Input: part model. Units: mm. Frame: model coordinates. A direction names the side the tool comes from. Coordinates: 2 decimals unless noted, no trailing zeros. Write each loop counter-clockwise with the first axis right and the second up, starting at its lowest first coordinate (ties: lowest second). Pieces come first, ordered by that corner, then holes. Notation, with made-up numbers: M 12.25,63.25 L 69.25,63.25 A20 ccw 69.25,70.25 Z; hole C 61.5,-2 d10. An arc over 180 degrees is marked long. Write each question's results on one line, items separated by ' | '. Start each with the question number.
1. First-contact query: pin 1 (10 mm diameter, centred on y = -29, z = 8, fed in from +X); pin 2 (5 mm diameter, centred on y = -5, z = 15.5, fed in from -X); pin 3 (4.5 mm diameter, centred on y = -5, z = -15.5, fed in from +X); pin 4 (14.5 mm diameter, centred on x = 0, z = 0, fed in from +Y). Flat tips, straight axial feed; report the tip coordinate or a pass-through.
2. Section query A-A, the plane y = 2.5. Count the separate pieces of the cut face and the enclosed holes in it, and give its area (3 significant figures).
3. Section query C-C, the plane y = -27. Output: boundary loops of the cut face in (x, z), and give its area (3 significant figures).
4. Section query B-B, the plane z = -6.5. Output: boundary loops of the cut face in (x, y), and give its area (3 significant figures).
5. Set-up query: faces 5 (the flat face through (-23.85, -30, -15)), 6 (the cylindrical face through (-24.8, -26.5, -14.7)). Return all of +Z, -Z, +X, -X, +Y, -Y with unobstructed straight access to the full face (end or side cutting, diameter ignored); none if empty.
6. Pull-direction query (Y, two-part tool) for faces 1 (the flat face through (-13, 5, 0)), 2 (the flat face through (-2.73, -16.6, -23.96)), 3 (the flat face through (-23.85, -5, -17.5)), 4 (the flat face through (-21, -16, 0)); classes: +Y half, -Y half, draft (parallel to the pull), parting line (faces both ways), or undercut.
7. Section query D-D, the plane x = 0. Output: boundary loops of the cut face in (y, z).
8. Ray query, probe 1 along Y at (x, z) = (-24.9, -15.5); probe 2 along Y at (x, z) = (-24, -15); probe 3 along Z at (x, y) = (-14.5, -12). Return the intervals inside material, ascending.
```python
from build123d import *

# Parameters (mm, degrees)
SKETCH1_R                = 12
SKETCH1_R_2              = 1.7
BOSS_EXTRUDE1_DEPTH      = 5
BOSS_EXTRUDE3_DEPTH      = 5
BOSS_EXTRUDE4_DEPTH      = 5
CHAMFER1_SIZE            = 5
CHAMFER1_OF_MIRROR1_SIZE = 5
SKETCH7_R                = 3
CUT_EXTRUDE1_DEPTH       = 3.1
CUT_EXTRUDE2_DEPTH       = 33.001420077


# Read off the part's stored shape, not the designer's step: Cut-Extrude2
with BuildPart() as part:
    # Sketch1 → Boss-Extrude1 (new body)
    with BuildSketch(Plane(origin=(0, 0, 0), x_dir=(1, 0, 0), z_dir=(0, 1, 0))):
        Polygon((-20.75, 21.139640519), (-20.75, -21.139640519), (15.50680609, -21.139640519), (20.75, -15.896446609), (20.75, 15.896446609), (15.50680609, 21.139640519), align=None)
        with Locations(Location((0, 0, 0), (0, 0, 270))):
            Circle(SKETCH1_R, mode=Mode.SUBTRACT)
        with Locations(Location((15.5, 15.5, 0), (0, 0, 270))):
            Circle(SKETCH1_R_2, mode=Mode.SUBTRACT)
        with Locations(Location((-15.5, -15.5, 0), (0, 0, 270))):
            Circle(SKETCH1_R_2, mode=Mode.SUBTRACT)
        with Locations(Location((15.5, -15.5, 0), (0, 0, 270))):
            Circle(SKETCH1_R_2, mode=Mode.SUBTRACT)
        with Locations(Location((-15.5, 15.5, 0), (0, 0, 270))):
            Circle(SKETCH1_R_2, mode=Mode.SUBTRACT)
    extrude(amount=BOSS_EXTRUDE1_DEPTH)

    # Sketch3 → Boss-Extrude3 (add)
    with BuildSketch(Plane(origin=(-20.75, 0.364318818, 0), x_dir=(0, 0, 1), z_dir=(-1, 0, 0))):
        Polygon((-21.139640519, 4.635681182), (-21.139640519, 4.634261105), (-21.139640519, -0.364318818), (21.139640519, -0.364318818), (21.139640519, 4.634261105), (21.139640519, 4.635681182), align=None)
        with BuildLine():
            Line((21.139640519, -0.364318818), (-21.139640519, -0.364318818))
            Line((-21.139640519, -0.364318818), (-21.139640519, -5.366500535))
            Line((-21.139640519, -5.366500535), (-17.2, -5.366500535))
            ThreePointArc((-17.2, -5.366500535), (-15.5, -3.666500535), (-13.8, -5.366500535))
            Line((-13.8, -5.366500535), (13.8, -5.366500535))
            ThreePointArc((13.8, -5.366500535), (15.5, -3.666500535), (17.2, -5.366500535))
            Line((17.2, -5.366500535), (21.139640519, -5.366500535))
            Line((21.139640519, -5.366500535), (21.139640519, -0.364318818))
        make_face()
        with BuildLine():
            Line((-17.2, -5.366500535), (-21.139640519, -5.366500535))
            Line((-21.139640519, -5.366500535), (-21.139640519, -28.365738895))
            Line((-21.139640519, -28.365738895), (-17.2, -28.365738895))
            ThreePointArc((-17.2, -28.365738895), (-15.5, -26.665738895), (-13.8, -28.365738895))
            Line((-13.8, -28.365738895), (13.8, -28.365738895))
            ThreePointArc((13.8, -28.365738895), (15.5, -26.665738895), (17.2, -28.365738895))
            Line((17.2, -28.365738895), (21.139640519, -28.365738895))
            Line((21.139640519, -28.365738895), (21.139640519, -5.366500535))
            Line((21.139640519, -5.366500535), (17.2, -5.366500535))
            ThreePointArc((17.2, -5.366500535), (15.5, -7.066500535), (13.8, -5.366500535))
            Line((13.8, -5.366500535), (-13.8, -5.366500535))
            ThreePointArc((-13.8, -5.366500535), (-15.5, -7.066500535), (-17.2, -5.366500535))
        make_face()
        with BuildLine():
            Line((-17.2, -28.365738895), (-21.139640519, -28.365738895))
            Line((-21.139640519, -28.365738895), (-21.139640519, -33.365738895))
            Line((-21.139640519, -33.365738895), (21.139640519, -33.365738895))
            Line((21.139640519, -33.365738895), (21.139640519, -28.365738895))
            Line((21.139640519, -28.365738895), (17.2, -28.365738895))
            ThreePointArc((17.2, -28.365738895), (15.5, -30.065738895), (13.8, -28.365738895))
            Line((13.8, -28.365738895), (-13.8, -28.365738895))
            ThreePointArc((-13.8, -28.365738895), (-15.5, -30.065738895), (-17.2, -28.365738895))
        make_face()
    extrude(amount=BOSS_EXTRUDE3_DEPTH)

    # Sketch6 → Boss-Extrude4 (add)
    with BuildSketch(Plane(origin=(0, 0, -21.139640519), x_dir=(-1, 0, 0), z_dir=(0, 0, -1))):
        Polygon((-15.50680609, 0), (20.75, -33.001420077), (25.75, -33.001420077), (25.75, 5), (-15.50680609, 5), align=None)
    boss_extrude4 = extrude(amount=BOSS_EXTRUDE4_DEPTH)

    # Chamfer1
    chamfer1_edges = [part.edges().sort_by_distance(p)[0] for p in [
        (15.50680609, 2.5, -26.139640519),
    ]]
    chamfer(chamfer1_edges, length=CHAMFER1_SIZE - 0.0001)  # a hair under: the kernel refuses the full size

    # Mirror1: Boss-Extrude4 across plane
    add(boss_extrude4.mirror(Plane(origin=(0, 0, 0), x_dir=(1, 0, 0), z_dir=(0, 0, -1))))

    # Chamfer1 of Mirror1
    chamfer1_of_mirror1_edges = [part.edges().sort_by_distance(p)[0] for p in [
        (15.50680609, 2.5, 26.139640519),
    ]]
    chamfer(chamfer1_of_mirror1_edges, length=CHAMFER1_OF_MIRROR1_SIZE - 0.0001)  # a hair under: the kernel refuses the full size

    # Sketch7 → Cut-Extrude1 (cut)
    with BuildSketch(Plane(origin=(-20.75, 0, 0), x_dir=(0, 0, -1), z_dir=(1, 0, 0))):
        with Locations((-15.5, -5.002181717)):
            Circle(SKETCH7_R)
        with Locations((15.5, -5.002181717)):
            Circle(SKETCH7_R)
        with Locations((-15.5, -28.001420077)):
            Circle(SKETCH7_R)
        with Locations((15.5, -28.001420077)):
            Circle(SKETCH7_R)
    extrude(amount=-CUT_EXTRUDE1_DEPTH, mode=Mode.SUBTRACT)

    # Cut-Extrude2 outline → Cut-Extrude2 (cut)
    with BuildSketch(Plane.XZ):
        Polygon((-21, 21.846747301), (-21, -21.846747301), (17, -21.846747301), (17, -21.139640519), (-20.75, -21.139640519), (-20.75, 21.139640519), (17, 21.139640519), (17, 21.846747301), align=None)
    extrude(amount=CUT_EXTRUDE2_DEPTH, mode=Mode.SUBTRACT)


solid = part.part
```
Answer:
1) pin 1: x = -21 | pin 2: x = -25.75 | pin 3: x = -23.85 | pin 4: through
2) separate pieces: 1 | enclosed holes: 5 | area: 1,840 mm^2
3) outline: M -25.75,-26.14 L -14.16,-26.14 L -14.16,-21.85 L -21,-21.85 L -21,-18.33 L -23.85,-18.33 L -23.85,-16.87 L -25.75,-16.87 Z; M -25.75,-14.13 L -23.85,-14.13 L -23.85,-12.67 L -21,-12.67 L -21,12.67 L -23.85,12.67 L -23.85,14.13 L -25.75,14.13 Z; M -25.75,16.87 L -23.85,16.87 L -23.85,18.33 L -21,18.33 L -21,21.85 L -14.16,21.85 L -14.16,26.14 L -25.75,26.14 Z | area: 264 mm^2
4) outline: M -25.75,-33 L -21,-33 L -21,0 L -10.09,0 L -10.09,5 L -25.75,5 Z; M 10.09,0 L 20.75,0 L 20.75,5 L 10.09,5 Z | area: 288 mm^2
5) face 5: +X | face 6: +X, -X
6) face 1: +Y half | face 2: -Y half | face 3: undercut | face 4: draft
7) outline: M -14.11,-26.14 L 5,-26.14 L 5,-12 L 0,-12 L 0,-21.85 L -14.11,-21.85 Z; M -14.11,21.85 L 0,21.85 L 0,12 L 5,12 L 5,26.14 L -14.11,26.14 Z
8) probe 1: -33 to -29.7, -26.3 to -6.7, -3.3 to 5 | probe 2: -33 to -29.63, -26.38 to -6.63, -3.38 to 5 | probe 3: -26.14 to -21.85, 21.85 to 26.14
